Build history of the part. All positions in model axes, mm. Round coordinates to 2 decimals unless told otherwise and drop trailing zeros. Write each loop counter-clockwise with the first axis right and the second up, starting at its lowest first coordinate (ties: lowest second). Pieces come first, ordered by that corner, then holes.
from build123d import *

# Parameters (mm, degrees)
SKETCH1_R           = 85.5
SKETCH1_R_2         = 2.38125
BOSS_EXTRUDE1_DEPTH = 6.35
SKETCH6_R           = 62.865
CUT_EXTRUDE3_DEPTH  = 122.081883451


with BuildPart() as part:
    # Sketch1 → Boss-Extrude1 (new body)
    with BuildSketch(Plane.XY):
        Circle(SKETCH1_R)
        with Locations((0, 78.499999972)):
            Circle(SKETCH1_R_2, mode=Mode.SUBTRACT)
        with Locations((78.5, 0)):
            Circle(SKETCH1_R_2, mode=Mode.SUBTRACT)
        with Locations((2.8e-08, -78.5)):
            Circle(SKETCH1_R_2, mode=Mode.SUBTRACT)
        with Locations((-78.499999972, -2.8e-08)):
            Circle(SKETCH1_R_2, mode=Mode.SUBTRACT)
    extrude(amount=BOSS_EXTRUDE1_DEPTH)

    # Sketch6 → Cut-Extrude3 (cut, through all)
    with BuildSketch(Plane(origin=(0, 0, 0), x_dir=(-1, 0, 0), z_dir=(0, 0, -1))):
        Circle(SKETCH6_R)
    extrude(amount=-CUT_EXTRUDE3_DEPTH, mode=Mode.SUBTRACT)


solid = part.part
1) Slice it at C-C (y = -78.5). Write the cut outline in (x, z).
Results:
outline: (-33.88, 0) - (-2.38, 0) - (-2.38, 6.35) - (-33.88, 6.35) - close; (2.38, 0) - (33.88, 0) - (33.88, 6.35) - (2.38, 6.35) - close
2) Slice it at D-D (z = 2). Write the cut outline in (x, y) (1 decimal).
Results:
outline: circle Ø171 at (0, 0); hole circle Ø4.8 at (-78.5, 0); hole circle Ø125.7 at (0, 0); hole circle Ø4.8 at (0, -78.5); hole circle Ø4.8 at (0, 78.5); hole circle Ø4.8 at (78.5, 0)
3) Slice it at A-A (x = 0). Write the cut outline in (y, z) (3 decimals).
Results:
outline: (-85.5, 0) - (-80.881, 0) - (-80.881, 6.35) - (-85.5, 6.35) - close; (-76.119, 0) - (-62.865, 0) - (-62.865, 6.35) - (-76.119, 6.35) - close; (62.865, 0) - (76.119, 0) - (76.119, 6.35) - (62.865, 6.35) - close; (80.881, 0) - (85.5, 0) - (85.5, 6.35) - (80.881, 6.35) - close
4) Pin check, flat tips, straight feed: pin 1 Ø3 at (x, z) = (-33, 3) entering from +Y; pin 2 Ø3 at (y, z) = (-14.5, 2.5) entering from +X; pin 3 Ø3 at (y, z) = (-63.5, 3.5) entering from +X. Stop position of each tip, or through.
Results:
pin 1: stops at y = 79.49
pin 2: stops at x = 84.51
pin 3: stops at x = 58.87
5) Wall check: L1, parallel to Y at x = 0, z = 2.25 (3 decimals); L2, parallel to X at y = -1.5, z = 1.75; L3, parallel to Y at x = -22, z = 1.75. Give the ranges that are in metal, low to high.
Results:
L1: y = -85.5 to -80.881, -76.119 to -62.865, 62.865 to 76.119, 80.881 to 85.5
L2: x = -85.49 to -80.35, -76.65 to -62.85, 62.85 to 76.65, 80.35 to 85.49
L3: y = -82.62 to -58.89, 58.89 to 82.62
